Check sheet for the modelled part. Datum: model origin and axes. Units: mm. Face numbers are marked on the shaded views. A direction names the side the tool comes from. Give positions to 0.01 mm unless a question says otherwise; leave off trailing zeros. Order: outer loops, then holes, each group sorted by start corner. A loop starts at its lowest first (then second) coordinate and runs counter-clockwise, first axis right, second up.
from build123d import *

# Parameters (mm, degrees)
F1_DEPTH = 70
F2_R     = 8
F3_DEPTH = 10
F4_R     = 5
F5_DEPTH = 70.001
F6_SIZE  = 1


# Not quite as in the source:
# - a feature names something its author has since deleted; it is built from what else it names


with BuildPart() as f1:
    # F0 (on Right) → F1 (new body)
    with BuildSketch(Plane.YZ):
        Polygon((-25, 67.5), (-54, 67.5), (-54, -67.5), (-25, -67.5), (-25, -42.5), (25, -42.5), (25, -67.5), (54, -67.5), (54, 67.5), (25, 67.5), (25, 42.5), (-25, 42.5), align=None)
    extrude(amount=F1_DEPTH)

    # F2 (on face) → F3 (cut)
    with BuildSketch(Plane(origin=(0, 0, 0), x_dir=(0, -1, 0), z_dir=(-1, 0, 0))):
        with Locations((41.9203005731, 41.5)):
            Circle(F2_R)
        with Locations((-42.0796994269, 41.5)):
            Circle(F2_R)
        with Locations((41.9203005731, -52.5)):
            Circle(F2_R)
        with Locations((-42.0796994269, -52.5)):
            Circle(F2_R)
    extrude(amount=-F3_DEPTH, mode=Mode.SUBTRACT)

    # F4 (on face) → F5 (cut, through all)
    with BuildSketch(Plane(origin=(0, 0, 0), x_dir=(0, -1, 0), z_dir=(-1, 0, 0))):
        with Locations((-42.0796994269, 41.5)):
            Circle(F4_R)
        with Locations((41.9203005731, 41.5)):
            Circle(F4_R)
        with Locations((41.9203005731, -52.5)):
            Circle(F4_R)
        with Locations((-42.0796994269, -52.5)):
            Circle(F4_R)
    extrude(amount=-F5_DEPTH, mode=Mode.SUBTRACT)

    # F6
    f6_edges = [f1.edges().sort_by_distance(p)[0] for p in [
        (70, -39.5, 67.5),
        (70, -25, 55),
        (70, -54, 0),
        (70, 0, 42.5),
        (70, -39.5, -67.5),
        (70, 25, 55),
        (70, -25, -55),
        (70, 39.5, 67.5),
        (70, 0, -42.5),
        (70, 54, 0),
        (70, 25, -55),
        (70, 39.5, -67.5),
        (70, -36.920301, -52.5),
        (70, 47.079699, -52.5),
        (70, -36.920301, 41.5),
        (70, 47.079699, 41.5),
        (35, -54, -67.5),
        (35, -25, -67.5),
        (35, 25, -67.5),
        (35, 54, -67.5),
        (35, -54, 67.5),
        (35, -25, 67.5),
        (35, 25, 67.5),
        (35, 54, 67.5),
    ]]
    chamfer(f6_edges, length=F6_SIZE)


solid = f1.part
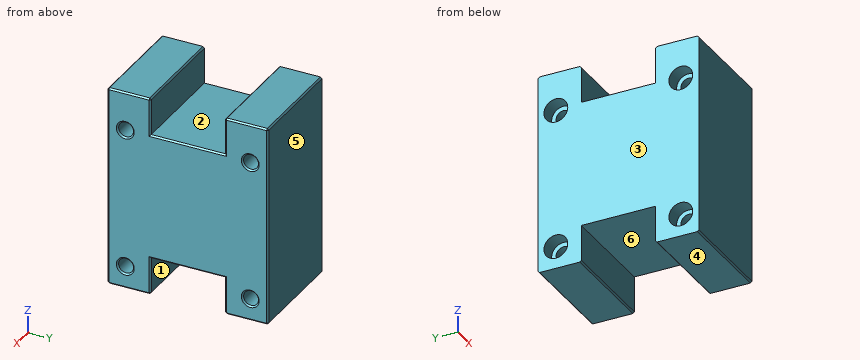
1) Set-up check for the marked faces 1, 2 and 3: record each of +Z, -Z, +X, -X, +Y, -Y from which the full face is reachable in a straight line by a thin tool's end or side.
Recorded:
face 1: -Z, +X, -X
face 2: +Z, +X, -X
face 3: +Z, -Z, -X, +Y, -Y
2) Section check D-D, the plane y = -4. Record the cut outline in (x, z), then the cut area to 3 significant figures.
Recorded:
outline: (0, -42.5) - (69, -42.5) - (70, -41.5) - (70, 41.5) - (69, 42.5) - (0, 42.5) - close
area: 5,950 mm2
3) Material ranges on L1, parallel to Y at x = 7, z = -52; L2, parallel to Z at x = 11.5, y = 42; L3, parallel to Y at x = 32, z = 41, recorded low to high.
Recorded:
L1: y = -54 to -49.9, -33.94 to -25, 25 to 34.1, 50.06 to 54
L2: z = -67.5 to -57.5, -47.5 to 36.5, 46.5 to 67.5
L3: y = -54 to -46.9, -36.95 to 37.1, 47.05 to 54
4) Draft check along Y on the marked faces 4, 5 and 6. Enter one of: +Y half, -Y half, draft (parallel to the pull), parting line (faces both ways), or undercut.
Recorded:
face 4: draft
face 5: +Y half
face 6: undercut
5) Section check B-B, the plane z = -52.5. State how many separate pieces and enclosed holes the cut face has, then the cut area to 3 significant figures.
Recorded:
separate pieces: 4
enclosed holes: 0
area: 2,540 mm2
6) Section check C-C, the plane z = 55.5. Record the cut outline in (x, y), then the cut area to 3 significant figures.
Recorded:
outline: (0, -54) - (69, -54) - (70, -53) - (70, -26) - (69, -25) - (0, -25) - close; (0, 25) - (69, 25) - (70, 26) - (70, 53) - (69, 54) - (0, 54) - close
area: 4,060 mm2
7) Depth check by flat-ended pin: pin 1 Ø13 at (y, z) = (-41.92, -52.5) entering from -X; pin 2 Ø3 at (x, y) = (10.5, -6.5) entering from +Z; pin 3 Ø11.5 at (y, z) = (42.08, 41.5) entering from +X. Enter the tip coordinate at first touch or a pass-through.
Recorded:
pin 1: stops at x = 10
pin 2: stops at z = 42.5
pin 3: stops at x = 69.75
8) Section check A-A, the plane x = 5.5. Record the cut outline in (y, z), then the cut area to 3 significant figures.
Recorded:
outline: (-54, -66.5) - (-53, -67.5) - (-26, -67.5) - (-25, -66.5) - (-25, -42.5) - (25, -42.5) - (25, -66.5) - (26, -67.5) - (53, -67.5) - (54, -66.5) - (54, 66.5) - (53, 67.5) - (26, 67.5) - (25, 66.5) - (25, 42.5) - (-25, 42.5) - (-25, 66.5) - (-26, 67.5) - (-53, 67.5) - (-54, 66.5) - close; hole circle Ø16 at (-41.92, -52.5); hole circle Ø16 at (-41.92, 41.5); hole circle Ø16 at (42.08, -52.5); hole circle Ø16 at (42.08, 41.5)
area: 11,300 mm2
